Geometry: final body of the model. Coordinates: model frame, mm. Face numbers are marked on the shaded views. A direction names the side the tool comes from. Round coordinates to 2 decimals unless told otherwise and drop trailing zeros. Loops run counter-clockwise (first coordinate to the right, second up) from the corner with the lowest first, then second, coordinate; pieces in that order, holes last. Notation, with made-up numbers: M 44,52.25 L 81,52.25 A24 cw 81,68.25 Z; hole C -18.5,59.5 d5. An arc over 180 degrees is marked long. Write each question's results on one line, items separated by ' | '.
Solid Edge part; units mm, degrees
sketch "Sketch1" plane through (0, 0, 0) normal (0, -1, 0) x (1, 0, 0)
  line L0 (6, 24) -> (12, 30)
  line L1 (0, 30) -> (12, 30)
  line L2 (0, 0) -> (0, 30)
  line L3 (0, 0) -> (6, 0)
  line L4 (6, 0) -> (6, 24)
revolve "RevolvedProtrusion1" add sketch "Sketch1" angle 360 about axis through (0, 0, 0) along (0, 0, 1)
cosmetic_thread "Thread1"
chamfer "Chamfer1" distance 0.5 angle 45 1 edges at (-6, 0, 0)
sketch "Sketch2" plane through (0, 0, 30) normal (0, 0, 1) x (1, 0, 0)
  line L0 (-1, 12) -> (-1, -12)
  line L1 (-1, -12) -> (1, -12)
  line L2 (1, -12) -> (1, 12)
  line L3 (1, 12) -> (-1, 12)
extrude "ExtrudedCutout_1" cut sketch "Sketch2" along normal mid plane 3
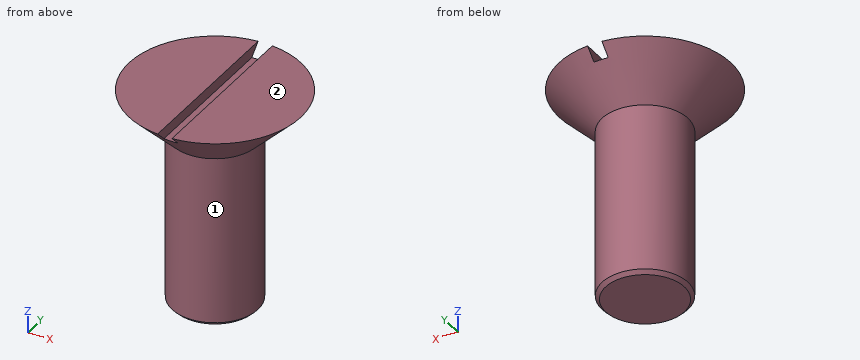
1. Section B-B (y = 0). Output: boundary loops of the cut face in (x, z).
Answer key:
outline: M -12,30 L -6,24 L -6,0.5 L -5.5,0 L 5.5,0 L 6,0.5 L 6,24 L 12,30 L 1,30 L 1,28.5 L -1,28.5 L -1,30 Z
2. Section C-C (z = 11). Output: boundary loops of the cut face in (x, y).
Answer key:
outline: C 0,0 d12
3. Access query for the marked faces 1 and 2. Directions: +Z, -Z, +X, -X, +Y, -Y. A direction counts if a zero-diameter tool reaches every point of the face in a straight line with its end or side. Return the directions, or none.
Answer key:
face 1: -Z | face 2: +Z, +X, -X, +Y, -Y
4. Pin query (flat end, axial travel): P1, Ø1.5, axis at x = 0.5, z = 5.5, coming from the -Y side; P2, Ø6, axis at y = 2, z = 21, coming from the -X side; P3, Ø2, axis at y = -2, z = 7.5, coming from the -X side; P4, Ø3, axis at x = 8, z = 21, coming from the +Y side. Return the tip coordinate at first contact, or that it passes through.
Answer key:
P1: stops at y = -6 | P2: stops at x = -6 | P3: stops at x = -5.92 | P4: passes through
5. Section A-A (x = 0). Output: boundary loops of the cut face in (y, z).
Answer key:
outline: M -10.5,28.5 L -6,24 L -6,0.5 L -5.5,0 L 5.5,0 L 6,0.5 L 6,24 L 10.5,28.5 Z
6. Ray query, probe 1 along X at (y, z) = (8.5, 29.5); probe 2 along Z at (x, y) = (0.5, -1.75); probe 3 along Z at (x, y) = (-2.75, 9). Return the intervals inside material, ascending.
Answer key:
probe 1: x = -7.75 to -1, 1 to 7.75 | probe 2: z = 0 to 28.5 | probe 3: z = 27.41 to 30
